The listing builds one solid part. Answer for the finished solid, in the listing's coordinates (mm). A direction names the side the tool comes from. Round coordinates to 2 decimals unless told otherwise and drop trailing zeros. Order: outer loops, then holes, each group sorted by start corner. A loop starts at its lowest first (then second) coordinate and runs counter-clockwise, first axis right, second up. Notation, with made-up numbers: (-6.5, -18) -> (45.5, -18) arc R25 cw to (45.5, -5) -> close; hole circle Ø4 at (-37, 73.25). An arc over 180 degrees is marked (long way). Answer in a Markdown table with one row per item. Add a question column.
```python
from build123d import *

# Parameters (mm, degrees)
F0_W      = 40
F0_H      = 43
F0_W_2    = 36
F0_H_2    = 39
F1_DEPTH  = 1.5
F2_DEPTH  = 14
F3_W      = 2
F3_H      = 38
F4_DEPTH  = 8
F5_R      = 2.5
F6_W      = 20
F6_H      = 0.05
F6_H_2    = 1.45
F7_DEPTH  = 5
F8_W      = 2
F8_H      = 15
F9_DEPTH  = 25
F10_W     = 1.5
F10_H     = 5
F11_DEPTH = 50


with BuildPart() as f1:
    # F0 (on Top) → F1 (new body)
    with BuildSketch(Plane.XY):
        Rectangle(F0_W, F0_H)
        Rectangle(F0_W_2, F0_H_2, mode=Mode.SUBTRACT)
        Rectangle(F0_W_2, F0_H_2)
    extrude(amount=F1_DEPTH)

    # F0 (on Top) → F2 (join)
    with BuildSketch(Plane.XY):
        Rectangle(F0_W, F0_H)
        Rectangle(F0_W_2, F0_H_2, mode=Mode.SUBTRACT)
    extrude(amount=F2_DEPTH)

    # F3 (on face) → F4 (cut)
    with BuildSketch(Plane.XY.offset(14)):
        with Locations((-19, 0)):
            Rectangle(F3_W, F3_H)
    extrude(amount=-F4_DEPTH, mode=Mode.SUBTRACT)

    # F5
    f5_edges = [f1.edges().sort_by_distance(p)[0] for p in [
        (-20, -21.5, 7),
        (20, -21.5, 7),
        (20, 21.5, 7),
        (-20, 21.5, 7),
        (0, -21.5, 0),
        (20, 0, 0),
        (0, 21.5, 0),
    ]]
    fillet(f5_edges, radius=F5_R)

    # F6 (on face) → F7 (cut)
    with BuildSketch(Plane.XY.offset(14)):
        with Locations((0, 19.475)):
            Rectangle(F6_W, F6_H)
        with Locations((0, -19.475)):
            Rectangle(F6_W, F6_H)
        with Locations((0, -20.225)):
            Rectangle(F6_W, F6_H_2)
        with Locations((0, 20.225)):
            Rectangle(F6_W, F6_H_2)
    extrude(amount=-F7_DEPTH, mode=Mode.SUBTRACT)

    # F8 (on face) → F9 (cut)
    with BuildSketch(Plane.XY.offset(1.5)):
        with Locations((-14.7980369404, 9.9996174034)):
            Rectangle(F8_W, F8_H)
        with Locations((-14.7980369404, -9.9996174034)):
            Rectangle(F8_W, F8_H)
        with Locations((-10.5980369404, 9.9996174034)):
            Rectangle(F8_W, F8_H)
        with Locations((-10.5980369404, -9.9996174034)):
            Rectangle(F8_W, F8_H)
        with Locations((-6.3980369404, 9.9996174034)):
            Rectangle(F8_W, F8_H)
        with Locations((-6.3980369404, -9.9996174034)):
            Rectangle(F8_W, F8_H)
        with Locations((-2.1980369404, 9.9996174034)):
            Rectangle(F8_W, F8_H)
        with Locations((-2.1980369404, -9.9996174034)):
            Rectangle(F8_W, F8_H)
        with Locations((2.0019630596, 9.9996174034)):
            Rectangle(F8_W, F8_H)
        with Locations((2.0019630596, -9.9996174034)):
            Rectangle(F8_W, F8_H)
        with Locations((6.2019630596, 9.9996174034)):
            Rectangle(F8_W, F8_H)
        with Locations((6.2019630596, -9.9996174034)):
            Rectangle(F8_W, F8_H)
        with Locations((10.4019630596, 9.9996174034)):
            Rectangle(F8_W, F8_H)
        with Locations((10.4019630596, -9.9996174034)):
            Rectangle(F8_W, F8_H)
        with Locations((14.6019630596, 9.9996174034)):
            Rectangle(F8_W, F8_H)
        with Locations((14.6019630596, -9.9996174034)):
            Rectangle(F8_W, F8_H)
    extrude(amount=-F9_DEPTH, mode=Mode.SUBTRACT)

    # F10 (on face) → F11 (cut)
    with BuildSketch(Plane.XZ.offset(21.5)):
        with Locations((-15.9102423415, 6.201856127)):
            Rectangle(F10_W, F10_H)
        with Locations((-11.4102423415, 6.201856127)):
            Rectangle(F10_W, F10_H)
        with Locations((-6.9102423415, 6.201856127)):
            Rectangle(F10_W, F10_H)
        with Locations((-2.4102423415, 6.201856127)):
            Rectangle(F10_W, F10_H)
        with Locations((2.0897576585, 6.201856127)):
            Rectangle(F10_W, F10_H)
        with Locations((6.5897576585, 6.201856127)):
            Rectangle(F10_W, F10_H)
        with Locations((11.0897576585, 6.201856127)):
            Rectangle(F10_W, F10_H)
        with Locations((15.5897576585, 6.201856127)):
            Rectangle(F10_W, F10_H)
    extrude(amount=-F11_DEPTH, mode=Mode.SUBTRACT)


solid = f1.part
```
Item 1: For a pull along Z with two mould halves and no side action, classify faces 4 (the face through (2, -2.5, 1)), 5 (the face through (-3.16, -21, 6)) as released by +Z, released by -Z, zero draft, split by the parting line, or undercut.
Item 2: The part is cut by section A-A, the plane z = 12.75. Give the vertices of the cut face in (x, y), and give its area (3 significant figures).
Item 3: Flat-ended cylindrical pins translate along their axes: P1, Ø0.8, axis at x = 2.5, z = 1, coming from the +Y side (3 decimals); P2, Ø1.6, axis at y = -12.5, z = 0.5, coming from the +X side; P3, Ø1, axis at y = 20.5, z = 6, coming from the -X side. Find the tip coordinate at first contact, or state that the pin passes through.
Item 4: The part is cut by section C-C, the plane z = 5.5. State how many separate pieces and enclosed holes the cut face has, and give its area (3 significant figures).
Item 5: A tool of negligible diameter and unlimited length cuts with its end or side. For faces 1 (the face through (-6.16, -21, 6)), 2 (the face through (0, 19.5, 6)), 3 (the face through (-9.598, -10, 1)), from which of +Z, -Z, +X, -X, +Y, -Y can it reach the whole face along a straight path? Write none if from no direction.
Item 6: The part is cut by section B-B, the plane x = -13. Give the vertices of the cut face in (y, z), and give its area (3 significant figures).
Item 7: Find the intervals of material crossed by probe 1 along X at (y, z) = (6.5, 4.5); probe 2 along Y at (x, z) = (-10, 5.25); probe 3 along Y at (x, z) = (8, 12.25), in increasing order. Write a range as [from, to].
Resolved:
| question | item | result |
|---|---|---|
| 1 | face 4 | zero draft |
| 1 | face 5 | undercut |
| 2 | outline | (-20, -19) arc R2.5 ccw to (-17.5, -21.5) -> (17.5, -21.5) arc R2.5 ccw to (20, -19) -> (20, 19) arc R2.5 ccw to (17.5, 21.5) -> (-17.5, 21.5) arc R2.5 ccw to (-20, 19) -> (-18, 19) -> (-18, 19.5) -> (-10, 19.5) -> (-10, 20.95) -> (10, 20.95) -> (10, 19.5) -> (18, 19.5) -> (18, -19.5) -> (10, -19.5) -> (10, -20.95) -> (-10, -20.95) -> (-10, -19.5) -> (-18, -19.5) -> (-18, -19) -> close |
| 2 | area | 177 mm2 |
| 3 | P1 | y = 21.245 |
| 3 | P2 | x = 19.69 |
| 3 | P3 | x = -19.79 |
| 4 | separate pieces | 16 |
| 4 | enclosed holes | 0 |
| 4 | area | 263 mm2 |
| 5 | face 1 | +Y, -Y |
| 5 | face 2 | +Z |
| 5 | face 3 | +Z, -Z |
| 6 | outline | (-21.5, 2.5) arc R2.5 ccw to (-19, 0) -> (19, 0) arc R2.5 ccw to (21.5, 2.5) -> (21.5, 14) -> (19.5, 14) -> (19.5, 1.5) -> (-19.5, 1.5) -> (-19.5, 14) -> (-21.5, 14) -> close |
| 6 | area | 112 mm2 |
| 7 | probe 1 | [-20, -18], [18, 20] |
| 7 | probe 2 | [-21.5, -19.5], [19.5, 21.5] |
| 7 | probe 3 | [-21.5, -20.95], [20.95, 21.5] |
